Print and shaded views of the part. All mm, measured from the part's lowest x, y and z. Coordinates: 2 decimals unless noted, no trailing zeros. Loops run counter-clockwise (first coordinate to the right, second up) from the corner with the lowest first, then second, coordinate; pieces in that order, holes last.
1) Saw through at A-A, the plane y = 7.25. Write the cut outline in (x, z), and give its area (3 significant figures).
2) Wall check: line 1 along Z through (x, y) = (17, 8); line 2 along Z through (x, y) = (16.25, 9); line 3 along X through (y, z) = (1.75, 1.5). Give the ranges that are in metal, low to high.
3) Saw through at C-C, the plane z = 2.5. Write the cut outline in (x, y).
4) Saw through at B-B, the plane x = 17.25. Write the cut outline in (y, z), and give its area (3 significant figures).
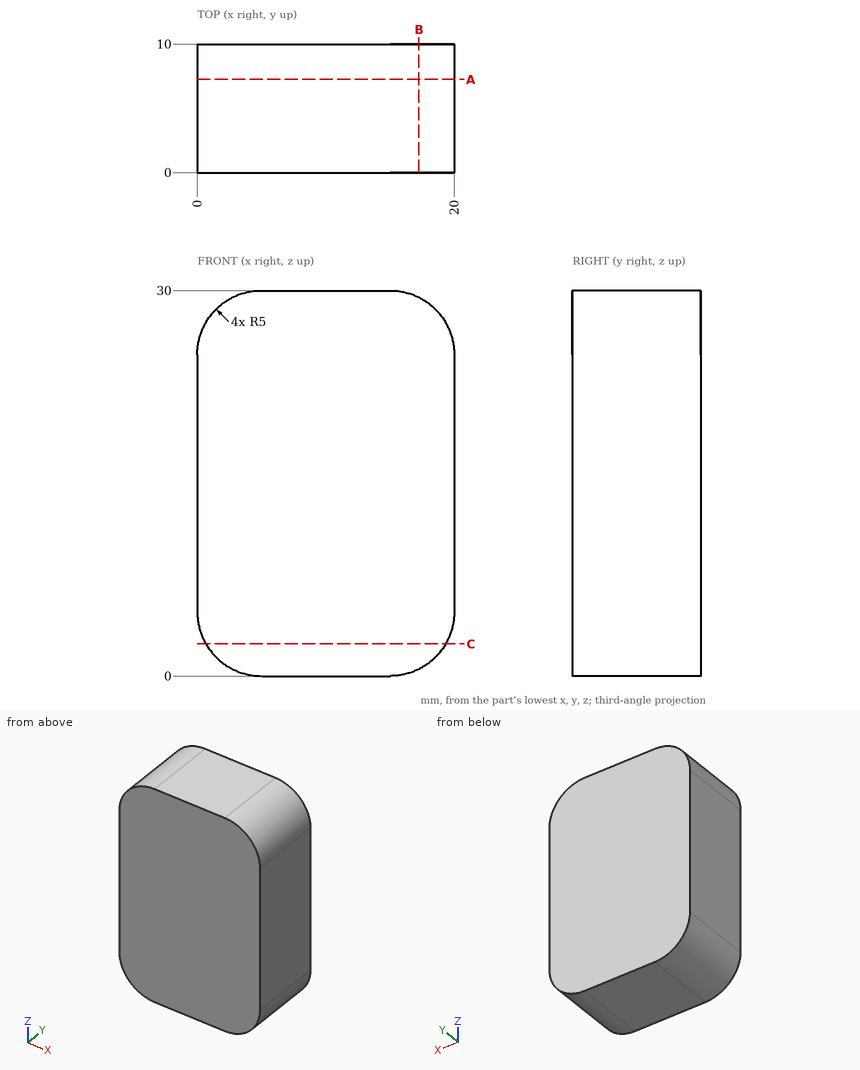
Data:
1. outline: (0, 5) arc R5 ccw to (5, 0) - (15, 0) arc R5 ccw to (20, 5) - (20, 25) arc R5 ccw to (15, 30) - (5, 30) arc R5 ccw to (0, 25) - close
1. area: 579 mm2
2. line 1: z = 0.42 to 29.58
2. line 2: z = 0.16 to 29.84
2. line 3: x = 1.43 to 18.57
3. outline: (0.67, 0) - (19.33, 0) - (19.33, 10) - (0.67, 10) - close
4. outline: (0, 0.53) - (10, 0.53) - (10, 29.47) - (0, 29.47) - close
4. area: 289 mm2
